Geometry: final body of the model. Coordinates: model frame, mm. Face numbers are marked on the shaded views. Give positions to 0.01 mm unless a question says otherwise; leave off trailing zeros. Write each loop counter-clockwise with the first axis right and the second up, starting at its lowest first coordinate (ties: lowest second). Pieces come first, ordered by that corner, then holes.
Q1. Pin query (flat end, axial travel): pin 1 Ø5 at (x, z) = (-22.31, 8.97) entering from +Y; pin 2 Ø6 at (x, z) = (-44, 5.5) entering from +Y; pin 3 Ø1.2 at (x, y) = (0.5, -59.5) entering from -Z; pin 4 Ø8 at (x, y) = (-43.5, -48) entering from +Z. Return the tip coordinate at first contact, or that it passes through.
Q2. Line query: line 1 (Y direction, x = -24, z = 2.75); line 2 (X direction, y = -69, z = 6.5); line 3 (Z direction, x = -53, y = -70.5). Output: solid intervals per line, ascending.
Q3. Section C-C (z = 8.25). Return the cut outline in (x, y).
Q4. Section B-B (y = -65). Return the cut outline in (x, z).
Q5. Mould query, pull axis Y, two halves, no side actions, for the marked faces 1, 2 and 3. Classes: +Y half, -Y half, draft (parallel to the pull), parting line (faces both ways), or undercut.
Q6. Section A-A (z = 11.25). Return the cut outline in (x, y).
Q7. Section D-D (x = -0.5). Return the cut outline in (y, z).
from build123d import *

# Parameters (mm, degrees)
BOX_W        = 50.8
BOX_H        = 12.7
BOX_DEPTH    = 12.7
PAD001_DEPTH = 4.064
SKETCH002_R  = 1.524
POCKET_DEPTH = 4.064
SKETCH_R     = 15.5
SKETCH_R_2   = 9.5
PAD_DEPTH    = 7.112


with BuildPart() as cube:
    # Box → Box (new body)
    with BuildSketch(Plane(origin=(-31.75, -63.5, 12.7), x_dir=(1, 0, 0), z_dir=(0, 0, 1))):
        with Locations((25.4, 6.35)):
            Rectangle(BOX_W, BOX_H)
    extrude(amount=BOX_DEPTH)


with BuildPart() as pocket:
    # Sketch001 → Pad001 (new body)
    with BuildSketch(Plane.XZ.offset(62.523445)):
        Polygon((-26.256083, 0.01423), (-26.256083, 25.000831), (-18.475065, 25.000831), (-18.475065, 4.985023), (5.922138, 4.985023), (5.922138, 25.000831), (13.703156, 25.000831), (13.703156, 0.01423), align=None)
    extrude(amount=-PAD001_DEPTH)

    # Sketch002 → Pocket (cut)
    with BuildSketch(Plane.XZ.offset(62.523445)):
        with Locations((-22.313841, 8.966419)):
            Circle(SKETCH002_R)
        with Locations((9.706401, 8.957657)):
            Circle(SKETCH002_R)
        Polygon((-21.182388, 22.588652), (-20.423353, 21.006459), (-21.197212, 19.431463), (-22.909247, 19.04623), (-24.284375, 20.136409), (-24.284375, 21.891251), (-22.896394, 22.965019), align=None)
        Polygon((10.823041, 22.583467), (11.583767, 20.99775), (10.808184, 19.419245), (9.092335, 19.033154), (7.714144, 20.125762), (7.714144, 21.884513), (9.105217, 22.960673), align=None)
    extrude(amount=-POCKET_DEPTH, mode=Mode.SUBTRACT)


with BuildPart() as cut:
    # Sketch → Pad (new body)
    with BuildSketch(Plane(origin=(-4.199891, 0, 2.6e-05), x_dir=(1, 0, -1e-06), z_dir=(-1e-06, 0, -1))):
        with Locations((-37.314136, 60.529943)):
            Circle(SKETCH_R)
        with Locations((-37.314136, 60.529943)):
            Circle(SKETCH_R_2, mode=Mode.SUBTRACT)
    extrude(amount=-PAD_DEPTH)

    # Fusion: union Pocket
    add(pocket.part)

    # Cut: cut Cube
    add(cube.part, mode=Mode.SUBTRACT)


solid = cut.part
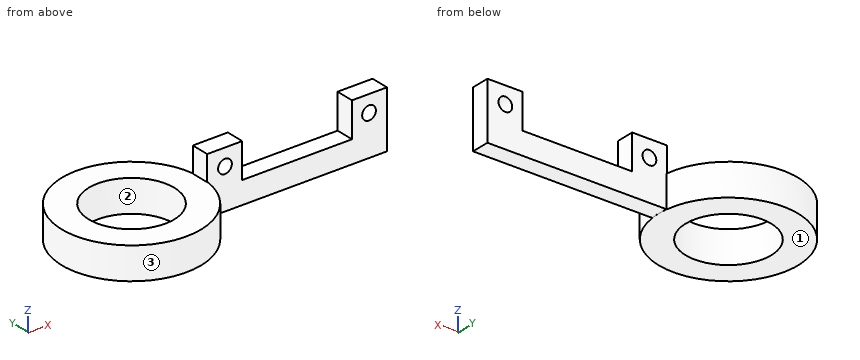
Computed:
1. pin 1: stops at y = -58.46
1. pin 2: stops at y = -45.03
1. pin 3: stops at z = 0.01
1. pin 4: stops at z = 7.11
2. line 1: y = -62.52 to -58.46
2. line 2: x = -54.5 to -45.82, -37.21 to -28.53
2. line 3: z = 0 to 7.11
3. outline: (-26.26, -62.52) - (-23.66, -62.52) - (-23.66, -58.46) - (-26.26, -58.46) - close; (-20.97, -62.52) - (-18.48, -62.52) - (-18.48, -58.46) - (-20.97, -58.46) - close; (5.92, -62.52) - (8.36, -62.52) - (8.36, -58.46) - (5.92, -58.46) - close; (11.06, -62.52) - (13.7, -62.52) - (13.7, -58.46) - (11.06, -58.46) - close
4. outline: (-56.36, 0) - (-49.9, 0) - (-49.9, 7.11) - (-56.36, 7.11) - close; (-33.13, 0) - (-26.67, 0) - (-26.67, 7.11) - (-33.13, 7.11) - close
5. face 1: draft
5. face 2: undercut
5. face 3: parting line
6. outline: (-26.26, -62.52) - (-18.48, -62.52) - (-18.48, -58.46) - (-26.26, -58.46) - close; (5.92, -62.52) - (13.7, -62.52) - (13.7, -58.46) - (5.92, -58.46) - close
7. outline: (-62.52, 0.01) - (-58.46, 0.01) - (-58.46, 4.99) - (-62.52, 4.99) - close
